Design review of the part built by this model. Coordinates are the model's own, in mm. Coordinates: 2 decimals unless noted, no trailing zeros. Write each loop counter-clockwise with the first axis right and the second up, starting at its lowest first coordinate (ties: lowest second). Pieces come first, ordered by that corner, then holes. Notation, with made-up numbers: (74.5, 20) - (110.5, 20) arc R22 ccw to (110.5, 49) - close; hole circle Ø5 at (63, 2). An arc over 180 degrees is marked (long way). One line per item, written item: value.
from build123d import *

# Parameters (mm, degrees)
F0_W     = 100
F0_H     = 100
F1_DEPTH = 100
F2_R     = 20
F3_SIZE  = 20
F4_R     = 15
F5_DEPTH = 100.001


with BuildPart() as f1:
    # F0 (on Front) → F1 (new body)
    with BuildSketch(Plane.XZ):
        Rectangle(F0_W, F0_H)
    extrude(amount=F1_DEPTH)

    # F2
    f2_edges = [f1.edges().sort_by_distance(p)[0] for p in [
        (-50, -50, 50),
        (50, -50, 50),
    ]]
    fillet(f2_edges, radius=F2_R)

    # F3
    f3_edges = [f1.edges().sort_by_distance(p)[0] for p in [
        (50, -50, -50),
        (-50, -50, -50),
    ]]
    chamfer(f3_edges, length=F3_SIZE)

    # F4 (on face) → F5 (cut, through all)
    with BuildSketch(Plane.XZ.offset(100)):
        Circle(F4_R)
    extrude(amount=-F5_DEPTH, mode=Mode.SUBTRACT)


solid = f1.part
1. Insertion check: pin 1 Ø5 at (x, y) = (38, -25) entering from +Z. The pin has a flat end and moves straight along its axis. Give the tip position at first contact, or say it passes through.
Answer block:
pin 1: stops at z = 49.23
2. Consider section D-D, the plane z = -43. Write out the cut boundary in (x, y), then the cut area to 3 significant figures.
Answer block:
outline: (-37, -100) - (37, -100) - (37, 0) - (-37, 0) - close
area: 7,400 mm^2
3. Consider section B-B, the plane x = -12. Write out the cut boundary in (y, z).
Answer block:
outline: (-100, -50) - (0, -50) - (0, -9) - (-100, -9) - close; (-100, 9) - (0, 9) - (0, 50) - (-100, 50) - close
4. Mouldability with a two-part tool opening along X and no side actions: class faces 1 (the face through (-14.985, -50.7, 0.66)), 2 (the face through (40, -49, -40)), 3 (the face through (-12, 0, 12)) as released by +X, released by -X, zero draft, split by the parting line, or undercut.
Answer block:
face 1: undercut
face 2: released by +X
face 3: zero draft
5. Wall thickness on line 1 along Z through (x, y) = (0, -52); line 2 along X through (y, z) = (-75, -6.5); line 3 along X through (y, z) = (-61, -9.5): over which ranges is each line inside the solid? List them lowest first.
Answer block:
line 1: z = -50 to -15, 15 to 50
line 2: x = -50 to -13.52, 13.52 to 50
line 3: x = -50 to -11.61, 11.61 to 50
6. Consider section C-C, the plane y = -46.5. Write out the cut boundary in (x, z), then the cut area to 3 significant figures.
Answer block:
outline: (-50, -30) - (-30, -50) - (30, -50) - (50, -30) - (50, 30) arc R20 ccw to (30, 50) - (-30, 50) arc R20 ccw to (-50, 30) - close; hole circle Ø30 at (0, 0)
area: 8,720 mm^2
7. Consider section A-A, the plane z = 0. Write out the cut boundary in (x, y).
Answer block:
outline: (-50, -100) - (-15, -100) - (-15, 0) - (-50, 0) - close; (15, -100) - (50, -100) - (50, 0) - (15, 0) - close
